Source: CAD feature listing. Evaluate the final solid. Frame: model axes, mm. Face numbers are marked on the shaded views. Coordinates: 2 decimals unless noted, no trailing zeros. Loops run counter-clockwise (first coordinate to the right, second up) from the corner with the lowest first, then second, coordinate; pieces in that order, holes last. Notation, with made-up numbers: M 21.25,-0.75 L 35.25,-0.75 A22 cw 35.25,8.25 Z; hole C 26.25,83.25 d3. An arc over 180 degrees is marked long. One line per question, with ' | ' between items. Start each with the question number.
1. Section query A-A, the plane x = -37.37. Output: boundary loops of the cut face in (y, z).
2. Section query B-B, the plane y = -16.69. Output: boundary loops of the cut face in (x, z).
3. Section query C-C, the plane z = 46.5. Output: boundary loops of the cut face in (x, y), and give its area (3 significant figures).
4. Ray query, probe 1 along Y at (x, z) = (-37.37, 49); probe 2 along X at (y, z) = (-16.75, 46); probe 3 along X at (y, z) = (-15.5, 47). Return the intervals inside material, ascending.
5. Pin query (flat end, axial travel): P1, Ø1, axis at y = -19.5, z = 47.5, coming from the +X side; P2, Ø3, axis at y = -14.5, z = 46, coming from the +X side; P3, Ø2, axis at y = -14, z = 49, coming from the -X side. Return the tip coordinate at first contact, or that it passes through.
6. Mould query, pull axis X, two halves, no side actions, for the marked faces 1, 2 and 3. Classes: pulls with the +X half, pulls with the -X half, needs draft (parallel to the pull), parting line crosses it, or undercut.
7. Section query D-D, the plane x = -34.75. Output: boundary loops of the cut face in (y, z), and give its area (3 significant figures).
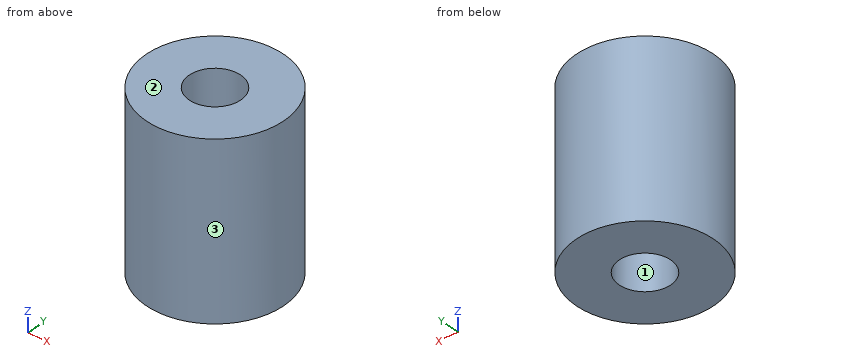
```python
from build123d import *

# Parameters (mm, degrees)
CYLINDER006_R     = 1.5
CYLINDER006_DEPTH = 10
CYLINDER007_R     = 4
CYLINDER007_DEPTH = 10


with BuildPart() as cylinder006:
    # Cylinder006 → Cylinder006 (new body)
    with BuildSketch(Plane(origin=(-37.37, -16.69, 44), x_dir=(1, 0, 0), z_dir=(0, 0, 1))):
        Circle(CYLINDER006_R)
    extrude(amount=CYLINDER006_DEPTH)


with BuildPart() as cut013014002:
    # Cylinder007 → Cylinder007 (new body)
    with BuildSketch(Plane(origin=(-37.37, -16.69, 44), x_dir=(1, 0, 0), z_dir=(0, 0, 1))):
        Circle(CYLINDER007_R)
    extrude(amount=CYLINDER007_DEPTH)

    # Cut013014002: cut Cylinder006
    add(cylinder006.part, mode=Mode.SUBTRACT)


solid = cut013014002.part
```
Taken from the geometry:
1) outline: M -20.69,44 L -18.19,44 L -18.19,54 L -20.69,54 Z; M -15.19,44 L -12.69,44 L -12.69,54 L -15.19,54 Z
2) outline: M -41.37,44 L -38.87,44 L -38.87,54 L -41.37,54 Z; M -35.87,44 L -33.37,44 L -33.37,54 L -35.87,54 Z
3) outline: C -37.37,-16.69 d8; hole C -37.37,-16.69 d3 | area: 43.2 mm^2
4) probe 1: -20.69 to -18.19, -15.19 to -12.69 | probe 2: -41.37 to -38.87, -35.87 to -33.37 | probe 3: -41.19 to -38.28, -36.46 to -33.55
5) P1: x = -34.1 | P2: x = -33.43 | P3: x = -41
6) face 1: undercut | face 2: needs draft | face 3: parting line crosses it
7) outline: M -19.71,44 L -13.67,44 L -13.67,54 L -19.71,54 Z | area: 60.5 mm^2
